```python
from build123d import *

# Parameters (mm, degrees)
EXTRUDE_1_DEPTH     = 2.5
EXTRUDE_2_DEPTH     = 9
SKETCH_6_W          = 14
SKETCH_6_H          = 8
SKETCH_6_W_2        = 9
SKETCH_6_H_2        = 5
CUT_EXTRUDE_3_DEPTH = 9
SKETCH_7_W          = 10
SKETCH_7_H          = 1.5
EXTRUDE_3_DEPTH     = 1
SKETCH_8_W          = 3
SKETCH_8_H          = 3
CUT_EXTRUDE_4_DEPTH = 5
EXTRUDE_4_DEPTH     = 2
SKETCH_10_W         = 15
SKETCH_10_H         = 1.883979019
EXTRUDE_5_DEPTH     = 4


with BuildPart() as part:
    # 草图1 → 凸台-拉伸1 (new body)
    with BuildSketch(Plane(origin=(0, 0, 0), x_dir=(1, 0, 0), z_dir=(0, 1, 0))):
        with BuildLine():
            Line((-32.5, 40), (32.5, 40))
            ThreePointArc((32.5, 40), (33.914213562, 39.414213562), (34.5, 38))
            Line((34.5, 38), (34.5, -38))
            ThreePointArc((34.5, -38), (33.914213562, -39.414213562), (32.5, -40))
            Line((32.5, -40), (-32.5, -40))
            ThreePointArc((-32.5, -40), (-33.914213562, -39.414213562), (-34.5, -38))
            Line((-34.5, -38), (-34.5, 38))
            ThreePointArc((-34.5, 38), (-33.914213562, 39.414213562), (-32.5, 40))
        make_face()
    extrude(amount=EXTRUDE_1_DEPTH)

    # 草图2 → 凸台-拉伸2 (add)
    with BuildSketch(Plane(origin=(0, 2.5, 0), x_dir=(1, 0, 0), z_dir=(0, 1, 0))):
        with BuildLine():
            Line((-32.5, -40), (32.5, -40))
            ThreePointArc((32.5, -40), (33.914213562, -39.414213562), (34.5, -38))
            Line((34.5, -38), (34.5, 38))
            ThreePointArc((34.5, 38), (33.914213562, 39.414213562), (32.5, 40))
            Line((32.5, 40), (-32.5, 40))
            ThreePointArc((-32.5, 40), (-33.914213562, 39.414213562), (-34.5, 38))
            Line((-34.5, 38), (-34.5, -38))
            ThreePointArc((-34.5, -38), (-33.914213562, -39.414213562), (-32.5, -40))
        make_face()
        with BuildLine():
            Line((-32.5, -38.5), (32.5, -38.5))
            ThreePointArc((32.5, -38.5), (32.853553391, -38.353553391), (33, -38))
            Line((33, -38), (33, 38))
            ThreePointArc((33, 38), (32.853553391, 38.353553391), (32.5, 38.5))
            Line((32.5, 38.5), (-32.5, 38.5))
            ThreePointArc((-32.5, 38.5), (-32.853553391, 38.353553391), (-33, 38))
            Line((-33, 38), (-33, -38))
            ThreePointArc((-33, -38), (-32.853553391, -38.353553391), (-32.5, -38.5))
        make_face(mode=Mode.SUBTRACT)
    extrude(amount=EXTRUDE_2_DEPTH)

    # 草图6 → 切除-拉伸3 (cut)
    with BuildSketch(Plane(origin=(0, 0, -40), x_dir=(-1, 0, 0), z_dir=(0, 0, -1))):
        with Locations((5.5, 6.5)):
            Rectangle(SKETCH_6_W, SKETCH_6_H)
        with Locations((-14, 5)):
            Rectangle(SKETCH_6_W_2, SKETCH_6_H_2)
    extrude(amount=-CUT_EXTRUDE_3_DEPTH, mode=Mode.SUBTRACT)

    # 草图7 → 凸台-拉伸3 (add)
    with BuildSketch(Plane(origin=(-33, 0, 0), x_dir=(0, 0, -1), z_dir=(1, 0, 0))):
        with Locations((33.771264053, 5.35)):
            Rectangle(SKETCH_7_W, SKETCH_7_H)
    extrude_3 = extrude(amount=EXTRUDE_3_DEPTH)

    # 镜向1: 凸台-拉伸3 across plane
    add(extrude_3.mirror(Plane(origin=(0, 0, 0), x_dir=(0, 0, 1), z_dir=(1, 0, 0))))

    # 草图8 → 切除-拉伸4 (cut)
    with BuildSketch(Plane(origin=(34.5, 0, 0), x_dir=(0, 0, -1), z_dir=(1, 0, 0))):
        with Locations((8.5, 10)):
            Rectangle(SKETCH_8_W, SKETCH_8_H)
        with Locations((-19.5, 10)):
            Rectangle(SKETCH_8_W, SKETCH_8_H)
    cut_extrude_4 = extrude(amount=-CUT_EXTRUDE_4_DEPTH, mode=Mode.SUBTRACT)

    # 镜向2: 切除-拉伸4 across plane
    add(cut_extrude_4.mirror(Plane(origin=(0, 0, 0), x_dir=(0, 0, 1), z_dir=(1, 0, 0))), mode=Mode.SUBTRACT)

    # 草图9 → 凸台-拉伸4 (add)
    with BuildSketch(Plane(origin=(0, 11.5, 0), x_dir=(1, 0, 0), z_dir=(0, 1, 0))):
        with BuildLine():
            Line((-34.5, 21), (34.5, 21))
            Line((34.5, 21), (34.5, 38))
            ThreePointArc((34.5, 38), (33.914213562, 39.414213562), (32.5, 40))
            Line((32.5, 40), (-32.5, 40))
            ThreePointArc((-32.5, 40), (-33.914213562, 39.414213562), (-34.5, 38))
            Line((-34.5, 38), (-34.5, 21))
        make_face()
    extrude(amount=EXTRUDE_4_DEPTH)

    # 草图10 → 凸台-拉伸5 (add)
    with BuildSketch(Plane(origin=(0, 2.5, 0), x_dir=(1, 0, 0), z_dir=(0, 1, 0))):
        with Locations((-25.5, -25.058010491)):
            Rectangle(SKETCH_10_W, SKETCH_10_H)
        with Locations((25.5, -25.058010491)):
            Rectangle(SKETCH_10_W, SKETCH_10_H)
    extrude(amount=EXTRUDE_5_DEPTH)


solid = part.part
```
Geometry check sheet. Reference: the model listing, model coordinates, mm. A direction names the side the tool comes from. Coordinates: 2 decimals unless noted, no trailing zeros. Order: outer loops, then holes, each group sorted by start corner. A loop starts at its lowest first (then second) coordinate and runs counter-clockwise, first axis right, second up.
Item 1: Scan lines: line 1 along Z through (x, y) = (-24, 9); line 2 along X through (y, z) = (8, -16); line 3 along Y through (x, z) = (-21, -30). Record each from-to range of solid material in increasing order.
Item 2: Tool access check on faces 4 (the flat face through (-26, 4, 24.116)), 5 (the flat face through (0, 11.5, 39)), 6 (the flat face through (18, 4, 25)), 7 (the flat face through (0, 11.5, -30)), 8 (the cylindrical face through (33.9, 5.67, 39.43)). Record the directions out of +Z, -Z, +X, -X, +Y, -Y that give a thin tool (end or side, any length) a straight path to the whole face; none if there is none.
Item 3: Section check A-A (z = -31). Enter the section's corners in (x, y), plus the area to 4 significant figures.
Item 4: Mould release check, pull along Y, two halves, no side actions. Record for faces 1 (the flat face through (0, 11, -38.5)), 2 (the flat face through (0, 0, -1)), 3 (the flat face through (-18, 4, 25)): released by +Y, released by -Y, zero draft, split by the parting line, or undercut.
Item 5: Depth check by flat-ended pin: pin 1 (0.8 mm diameter, centred on x = 33.5, z = 4.5, fed in from +Y); pin 2 (1.2 mm diameter, centred on x = -34, y = 10.5, fed in from +Z); pin 3 (5 mm diameter, centred on x = -4, z = 20, fed in from +Y). Enter the tip coordinate at first touch or a pass-through.
Item 6: Section check D-D (x = -23). Enter the section's corners in (y, z), plus the area to 3 significant figures.
Item 7: Section check B-B (x = 0.5). Enter the section's corners in (y, z).
Item 8: Section check C-C (z = 27.5). Enter the section's corners in (x, y), plus the area to 4 significant figures.
Check sheet entries:
1. line 1: z = -40 to -38.5, 38.5 to 40
1. line 2: x = -34.5 to -33, 33 to 34.5
1. line 3: y = 0 to 2.5, 11.5 to 13.5
2. face 4: +Y
2. face 5: +Z, +X, -X, +Y
2. face 6: -Z, +Y
2. face 7: none
2. face 8: +Z, +X, +Y, -Y
3. outline: (-34.5, 0) - (34.5, 0) - (34.5, 13.5) - (-34.5, 13.5) - close; hole (-33, 2.5) - (33, 2.5) - (33, 4.6) - (32, 4.6) - (32, 6.1) - (33, 6.1) - (33, 11.5) - (-33, 11.5) - (-33, 6.1) - (-32, 6.1) - (-32, 4.6) - (-33, 4.6) - close
3. area: 340.5 mm2
4. face 1: undercut
4. face 2: released by -Y
4. face 3: zero draft
5. pin 1: stops at y = 11.5
5. pin 2: stops at z = 39.79
5. pin 3: stops at y = 2.5
6. outline: (0, -40) - (13.5, -40) - (13.5, -21) - (11.5, -21) - (11.5, -38.5) - (2.5, -38.5) - (2.5, 24.12) - (6.5, 24.12) - (6.5, 26) - (2.5, 26) - (2.5, 38.5) - (11.5, 38.5) - (11.5, 40) - (0, 40) - close
6. area: 273 mm2
7. outline: (0, -40) - (2.5, -40) - (2.5, 38.5) - (11.5, 38.5) - (11.5, 40) - (0, 40) - close; (10.5, -40) - (13.5, -40) - (13.5, -21) - (11.5, -21) - (11.5, -38.5) - (10.5, -38.5) - close
8. outline: (-34.5, 0) - (34.5, 0) - (34.5, 11.5) - (33, 11.5) - (33, 2.5) - (-33, 2.5) - (-33, 11.5) - (-34.5, 11.5) - close
8. area: 199.5 mm2
